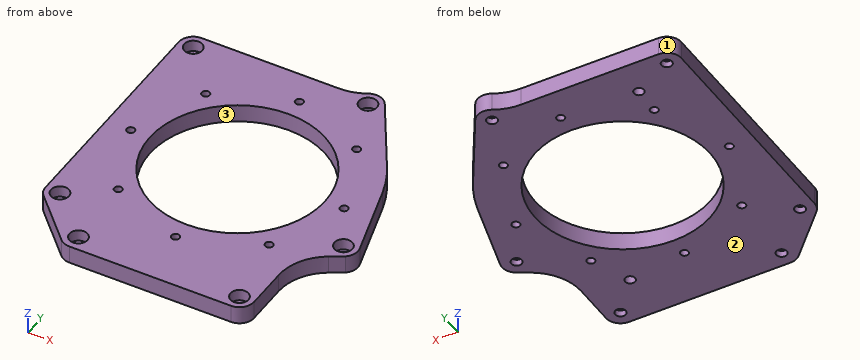
from build123d import *

# Parameters (mm, degrees)
BOSS_EXTRUDE1_DEPTH             = 18.0086
FILLET2_R                       = 50.8
CBORE_FOR_M10_SHCS7_D           = 10.5
CBORE_FOR_M10_SHCS7_CBORE_D     = 18
CBORE_FOR_M10_SHCS7_CBORE_DEPTH = 11.5
F_10_0MM_DOWEL_HOLE3_D          = 10
F_10_0MM_DOWEL_HOLE3_DEPTH      = 10
F_10_0MM_DOWEL_HOLE3_TIP        = 3.004303095
SKETCH79_R                      = 87.5
CUT_EXTRUDE3_DEPTH              = 221.734456483
F_3_8_16_TAPPED_HOLE3_D         = 7.9375


with BuildPart() as part:
    # Sketch1 → Boss-Extrude1 (new body)
    with BuildSketch(Plane.XY):
        with BuildLine():
            Line((103.452131625, -149.547952394), (103.452131625, -78.357146561))
            Line((103.452131625, -78.357146561), (140.546655396, -56.14120472))
            ThreePointArc((140.546655396, -56.14120472), (145.621790531, -49.117452101), (145.848381407, -40.454960885))
            Line((145.848381407, -40.454960885), (124.68673049, 34.942398048))
            ThreePointArc((124.68673049, 34.942398048), (117.704280966, 53.953895974), (107.843572082, 71.644517079))
            Line((107.843572082, 71.644517079), (65.450124697, 141.120289253))
            ThreePointArc((65.450124697, 141.120289253), (56.413981198, 147.677287258), (45.396832362, 145.869375848))
            Line((45.396832362, 145.869375848), (35.245747779, 139.53567106))
            Line((35.245747779, 139.53567106), (-116.713297339, 139.53567106))
            ThreePointArc((-116.713297339, 139.53567106), (-126.966345666, 135.288719387), (-131.213297339, 125.03567106))
            Line((-131.213297339, 125.03567106), (-131.213297339, -104.964264785))
            ThreePointArc((-131.213297339, -104.964264785), (-130.122475458, -110.515726026), (-127.012211231, -115.241704308))
            Line((-127.012211231, -115.241704308), (-83.421786595, -159.651825232))
            ThreePointArc((-83.421786595, -159.651825232), (-78.439848506, -163.031227751), (-72.538298924, -164.219411681))
            Line((-72.538298924, -164.219411681), (88.682165599, -164.219411681))
            ThreePointArc((88.682165599, -164.219411681), (99.120094961, -159.957126401), (103.452131625, -149.547952394))
        make_face()
    extrude(amount=BOSS_EXTRUDE1_DEPTH)

    # Fillet2
    fillet2_edges = [part.edges().sort_by_distance(p)[0] for p in [
        (35.245747779, 139.53567106, 9.0043),
        (103.452131625, -78.357146561, 9.0043),
    ]]
    fillet(fillet2_edges, radius=FILLET2_R)

    # CBORE for M10 SHCS7 (through all)
    with Locations(Plane.XY.offset(18.0086)):
        with Locations((-116.713297339, 125.03567106), (-116.541509562, -104.964264785), (-72.538298924, -148.969218673), (53.072470058, 133.567563544), (131.722431635, -44.419667636), (88.780343848, -149.547952394)):
            CounterBoreHole(CBORE_FOR_M10_SHCS7_D / 2, CBORE_FOR_M10_SHCS7_CBORE_D / 2, CBORE_FOR_M10_SHCS7_CBORE_DEPTH)

    # Ø10.0mm Dowel Hole3
    with Locations(Plane(origin=(0, 0, 0), x_dir=(-1, 0, 0), z_dir=(0, 0, -1))):
        with Locations((76.55340813, 103.753913834), (-59.102558089, -114.980445858)):
            Hole(F_10_0MM_DOWEL_HOLE3_D / 2, depth=F_10_0MM_DOWEL_HOLE3_DEPTH)
            with Locations((0, 0, -(F_10_0MM_DOWEL_HOLE3_DEPTH + F_10_0MM_DOWEL_HOLE3_TIP / 2))):  # 118° drill point
                Cone(0, F_10_0MM_DOWEL_HOLE3_D / 2, F_10_0MM_DOWEL_HOLE3_TIP, mode=Mode.SUBTRACT)

    # Sketch79 → Cut-Extrude3 (cut, through all)
    with BuildSketch(Plane.XY.offset(18.0086)):
        Circle(SKETCH79_R)
    extrude(amount=-CUT_EXTRUDE3_DEPTH, mode=Mode.SUBTRACT)

    # 3/8-16 Tapped Hole3 (through all)
    with Locations(Plane.XY.offset(18.0086)):
        with Locations((75.434151417, -75.434151417), (75.434151417, 75.434151417), (-75.434151417, 75.434151417), (-75.434151417, -75.434151417), (106.68, 0), (0, -106.68), (0, 106.68), (-106.68, 0)):
            Hole(F_3_8_16_TAPPED_HOLE3_D / 2)


solid = part.part
Work out the finished part from the listing and answer in its coordinate system (mm). Face numbers are marked on the shaded views. Coordinates: 2 decimals unless noted, no trailing zeros. Loops run counter-clockwise (first coordinate to the right, second up) from the corner with the lowest first, then second, coordinate; pieces in that order, holes last. Notation, with made-up numbers: M 7.25,-32 L 57.25,-32 A17 cw 57.25,-16 Z; hole C 9,31 d5. An arc over 180 degrees is marked long. Answer in a Markdown table with one row per item. Add a question column.
1. Find section B-B, the plane x = -41. Write down the section's boundary in (y, z).
2. Consider L1, parallel to Y at x = -0.5, z = 3.75; L2, parallel to Y at x = -72, z = 3.5; L3, parallel to Y at x = -2, z = 2.25. Determine where each line is inside the solid, lowest interval first.
3. Flat-ended cylindrical pins translate along their axes: P1, Ø4, axis at x = 25.5, z = 8.5, coming from the +Y side; P2, Ø6.5, axis at x = 88.78, y = -149.55, coming from the +Z side; P3, Ø10, axis at y = -1, z = 6.5, coming from the +X side; P4, Ø6, axis at y = 4, z = 13.5, coming from the +X side. Find the tip coordinate at first contact, or state that the pin passes through.
4. The mould has two halves that part along X. Classify the marked faces 1, 2 and 3: pulls with the +X half, pulls with the -X half, needs draft (parallel to the pull), parting line crosses it, or undercut.
5. Find section D-D, the plane z = 3. State how many separate pieces and enclosed holes the cut face has, then the cut area to 3 significant figures.
6. Find section A-A, the plane x = 0. Write down the section's boundary in (y, z).
7. Find section C-C, the plane y = -19.5. Write down the section's boundary in (x, z), then the cut area to 3 significant figures.
Reported:
| question | item | result |
|---|---|---|
| 1 | outline | M -164.22,0 L -77.3,0 L -77.3,18.01 L -164.22,18.01 Z; M 77.3,0 L 139.54,0 L 139.54,18.01 L 77.3,18.01 Z |
| 2 | L1 | y = -164.22 to -110.62, -102.74 to -87.5, 87.5 to 102.74, 110.62 to 139.54 |
| 2 | L2 | y = -164.22 to -154.19, -143.75 to -77.42, -73.44 to -49.72, 49.72 to 73.44, 77.42 to 101.69, 105.82 to 139.54 |
| 2 | L3 | y = -164.22 to -110.11, -103.25 to -87.48, 87.48 to 103.25, 110.11 to 139.54 |
| 3 | P1 | stops at y = 139.98 |
| 3 | P2 | passes through |
| 3 | P3 | stops at x = 136.18 |
| 3 | P4 | stops at x = 134.21 |
| 4 | face 1 | pulls with the -X half |
| 4 | face 2 | needs draft |
| 4 | face 3 | undercut |
| 5 | separate pieces | 1 |
| 5 | enclosed holes | 17 |
| 5 | area | 47,900 mm^2 |
| 6 | outline | M -164.22,0 L -110.65,0 L -110.65,18.01 L -164.22,18.01 Z; M -102.71,0 L -87.5,0 L -87.5,18.01 L -102.71,18.01 Z; M 87.5,0 L 102.71,0 L 102.71,18.01 L 87.5,18.01 Z; M 110.65,0 L 139.54,0 L 139.54,18.01 L 110.65,18.01 Z |
| 7 | outline | M -131.21,0 L -85.3,0 L -85.3,18.01 L -131.21,18.01 Z; M 85.3,0 L 139.97,0 L 139.97,18.01 L 85.3,18.01 Z |
| 7 | area | 1,810 mm^2 |
